Model file for the job. Use its own axes, mm. A direction names the side the tool comes from. Round coordinates to 2 decimals unless told otherwise and drop trailing zeros. Order: outer loops, then holes, each group sorted by start corner. A loop starts at its lowest first (then second) coordinate and runs counter-clockwise, first axis right, second up. Notation, with made-up numbers: (36.5, 85) - (48.5, 85) arc R13 cw to (48.5, 110) - close; hole circle Ø10 at (34.5, 4). An arc over 180 degrees is marked (long way). Use one line per item in the form item = value.
from build123d import *

# Parameters (mm, degrees)
ESQUISSE1_R        = 16
BOSS_EXTRU_1_DEPTH = 36
ESQUISSE2_R        = 18
BOSS_EXTRU_2_DEPTH = 70
CHANFREIN1_SIZE    = 2
ESQUISSE3_R        = 16
BOSS_EXTRU_3_DEPTH = 6
ESQUISSE4_R        = 14.5
BOSS_EXTRU_4_DEPTH = 18
CHANFREIN2_SIZE    = 1.5
ESQUISSE5_W        = 29
ESQUISSE5_H        = 18
BOSS_EXTRU_5_DEPTH = 25.5
ESQUISSE6_R        = 5.5
BOSS_EXTRU_6_DEPTH = 20


with BuildPart() as part:
    # Esquisse1 → Boss.-Extru.1 (new body)
    with BuildSketch(Plane(origin=(0, 0, 0), x_dir=(1, 0, 0), z_dir=(0, 1, 0))):
        with Locations(Location((0, 0, 0), (0, 0, 270))):
            Circle(ESQUISSE1_R)
    extrude(amount=BOSS_EXTRU_1_DEPTH)

    # Esquisse2 → Boss.-Extru.2 (add)
    with BuildSketch(Plane(origin=(0, 36, 0), x_dir=(1, 0, 0), z_dir=(0, 1, 0))):
        with Locations(Location((0, 0, 0), (0, 0, 270))):
            Circle(ESQUISSE2_R)
    extrude(amount=BOSS_EXTRU_2_DEPTH)

    # Chanfrein1
    chanfrein1_edges = [part.edges().sort_by_distance(p)[0] for p in [
        (0, 36, -18),
    ]]
    chamfer(chanfrein1_edges, length=CHANFREIN1_SIZE - 0.0001)  # a hair under: the kernel refuses the full size

    # Esquisse3 → Boss.-Extru.3 (add)
    with BuildSketch(Plane(origin=(0, 106, 0), x_dir=(1, 0, 0), z_dir=(0, 1, 0))):
        with Locations(Location((0, 0, 0), (0, 0, 270))):
            Circle(ESQUISSE3_R)
    extrude(amount=BOSS_EXTRU_3_DEPTH)

    # Esquisse4 → Boss.-Extru.4 (add)
    with BuildSketch(Plane(origin=(0, 112, 0), x_dir=(1, 0, 0), z_dir=(0, 1, 0))):
        with Locations(Location((0, 0, 0), (0, 0, 270))):
            Circle(ESQUISSE4_R)
    extrude(amount=BOSS_EXTRU_4_DEPTH)

    # Chanfrein2
    chanfrein2_edges = [part.edges().sort_by_distance(p)[0] for p in [
        (0, 112, -16),
    ]]
    chamfer(chanfrein2_edges, length=CHANFREIN2_SIZE - 0.0001)  # a hair under: the kernel refuses the full size

    # Esquisse5 → Boss.-Extru.5 (add)
    with BuildSketch(Plane.XY):
        with Locations((-0.063832193, 121)):
            Rectangle(ESQUISSE5_W, ESQUISSE5_H)
    extrude(amount=BOSS_EXTRU_5_DEPTH)

    # Esquisse6 → Boss.-Extru.6 (add)
    with BuildSketch(Plane.XZ):
        with Locations(Location((0, 0, 0), (0, 0, 90))):
            Circle(ESQUISSE6_R)
    extrude(amount=BOSS_EXTRU_6_DEPTH)


solid = part.part
(1) Slice it at A-A on y = 34.5. Give the cut face in (x, z), then the cut area to 3 significant figures.
Report:
outline = circle Ø32 at (0, 0)
area = 804 mm2
(2) Tool access for faces 4 (the face through (0, 0, 7)), 5 (the face through (-11, 106, -12)): list every direction of +Z, -Z, +X, -X, +Y, -Y with a clear straight run to the whole face (end or side of a thin tool).
Report:
face_4 = -Y
face_5 = none
(3) Slice it at C-C on y = 90. Give the cut face in (x, z).
Report:
outline = circle Ø36 at (0, 0)
(4) Slice it at B-B on z = 23.5. Give the cut face in (x, y), then the cut area to 3 significant figures.
Report:
outline = (-14.56, 112) - (14.44, 112) - (14.44, 130) - (-14.56, 130) - close
area = 522 mm2
(5) Pin check, flat tips, straight feed: pin 1 (9 mm diameter, centred on y = 121.5, z = 14, fed in from +X); pin 2 (8 mm diameter, centred on y = 92.5, z = 0.5, fed in from +X); pin 3 (10 mm diameter, centred on y = 59, z = 5, fed in from -X); pin 4 (12 mm diameter, centred on x = 2.5, y = 73, fed in from -Z). Stop position of each tip, or through.
Report:
pin_1 = 14.44
pin_2 = 18
pin_3 = -18
pin_4 = -18
(6) Probe probe 1 along Y at (x, z) = (0.5, 11); probe 2 along Y at (x, z) = (-10, 17); probe 3 along Y at (x, z) = (3, 14.5). List the from-to ranges inside material, lowest first. Write a range as [from, to].
Report:
probe_1 = [0, 130]
probe_2 = [112, 130]
probe_3 = [0, 111.69], [112, 130]
(7) Pull direction Y, two halves, no side cores. Call faces 1 (the face through (-15.62, 108.22, -3.47)), 2 (the face through (0, 130, 5)), 3 (the face through (-14.564, 121, 13)): released by +Y, released by -Y, zero draft, split by the parting line, or undercut.
Report:
face_1 = undercut
face_2 = released by +Y
face_3 = zero draft
